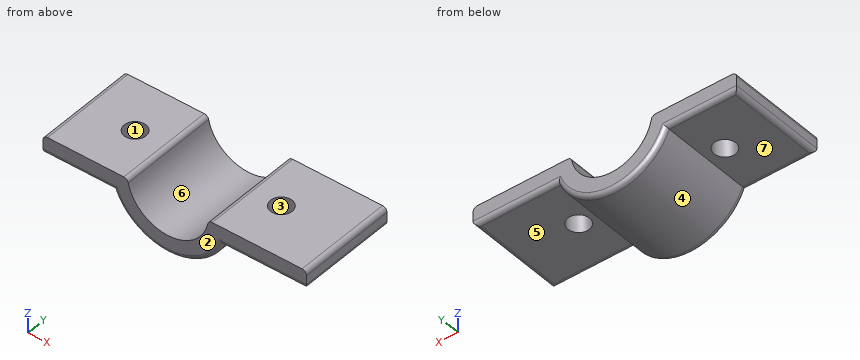
from build123d import *

# Parameters (mm, degrees)
BOSS_EXTRUDE1_DEPTH = 11
SKETCH2_R           = 1.2
CUT_EXTRUDE1_DEPTH  = 2
FILLET1_R           = 0.5


with BuildPart() as part:
    # Sketch1 → Boss-Extrude1 (new body)
    with BuildSketch(Plane(origin=(0, 0, 0), x_dir=(1, 0, 0), z_dir=(0, 1, 0))):
        with BuildLine():
            Line((6, 2.5), (15.35, 2.5))
            Line((15.35, 2.5), (15.35, 0.5))
            Line((15.35, 0.5), (6.480740698, 0.5))
            Line((6.480740698, 0.5), (4.472135955, 0.5))
            ThreePointArc((4.472135955, 0.5), (0, 4.5), (-4.472135955, 0.5))
            Line((-4.472135955, 0.5), (-6.480740698, 0.5))
            Line((-6.480740698, 0.5), (-13.85, 0.5))
            Line((-13.85, 0.5), (-13.85, 2.5))
            Line((-13.85, 2.5), (-6, 2.5))
            ThreePointArc((-6, 2.5), (0, 6.5), (6, 2.5))
        make_face()
    extrude(amount=BOSS_EXTRUDE1_DEPTH)

    # Sketch2 → Cut-Extrude1 (cut)
    with BuildSketch(Plane(origin=(0, 0, -2.5), x_dir=(-1, 0, 0), z_dir=(0, 0, -1))):
        with Locations((-8.1, 5.5)):
            Circle(SKETCH2_R)
        with Locations((8.1, 5.5)):
            Circle(SKETCH2_R)
    extrude(amount=-CUT_EXTRUDE1_DEPTH, mode=Mode.SUBTRACT)

    # Fillet1
    fillet1_edges = [part.edges().sort_by_distance(p)[0] for p in [
        (0, 11, -6.5),
        (-9.925, 0, -2.5),
        (0, 0, -6.5),
        (10.675, 0, -2.5),
        (-9.925, 11, -2.5),
        (15.35, 5.5, -2.5),
        (15.35, 5.5, -0.5),
        (4.472135955, 5.5, -0.5),
        (-4.472135955, 5.5, -0.5),
        (-13.85, 5.5, -0.5),
        (-13.85, 5.5, -2.5),
        (10.675, 11, -2.5),
    ]]
    fillet(fillet1_edges, radius=FILLET1_R)


solid = part.part
Can you work these out from the model? Positions are in its coordinate system, mm. Face numbers are marked on the shaded views. A direction names the side the tool comes from. Round coordinates to 2 decimals unless told otherwise and drop trailing zeros. Order: outer loops, then holes, each group sorted by start corner. A loop starts at its lowest first (then second) coordinate and runs counter-clockwise, first axis right, second up. Notation, with made-up numbers: (12.25, 72.5) - (59.25, 72.5) arc R13 ccw to (59.25, 82.5) - close; hole circle Ø3 at (8, 3.5). An arc over 180 degrees is marked (long way). Answer in a Markdown table with one row per item.
(1) Suppose I cut it at B-B, the plane x = 8.1. Please give me the cut outline in (y, z), plus the area to 3 significant figures.
From the geometry:
| item | result |
|---|---|
| outline | (0, -2) arc R0.5 ccw to (0.5, -2.5) - (4.3, -2.5) - (4.3, -0.5) - (0, -0.5) - close; (6.7, -2.5) - (10.5, -2.5) arc R0.5 ccw to (11, -2) - (11, -0.5) - (6.7, -0.5) - close |
| area | 17.1 mm2 |
(2) For P1, Ø3, axis at x = -8.1, y = 5.5, coming from the +Z side; P2, Ø6, axis at x = -11.5, y = 5, coming from the -Z side; P3, Ø2, axis at y = 8, z = -4, coming from the +X side; P4, Ø2, axis at x = 12.5, z = -5, coming from the -Y side, each with a flat end and sliding along its axis, tell me the tip position at first contact or that it passes through.
From the geometry:
| item | result |
|---|---|
| P1 | stops at z = -0.5 |
| P2 | stops at z = -2.5 |
| P3 | stops at x = 5.77 |
| P4 | passes through |
(3) Please list where these lines run through material, in increasing order: L1, parallel to Y at x = -8.1, z = -1.1; L2, parallel to Z at x = 9.75, y = 3.5; L3, parallel to X at y = 3.75, z = -2.75. Write a range as from..to.
From the geometry:
| item | result |
|---|---|
| L1 | y = 0..4.3, 6.7..11 |
| L2 | z = -2.5..-0.5 |
| L3 | x = -5.89..-3.56, 3.56..5.89 |
(4) Which directions (+Z, -Z, +X, -X, +Y, -Y) give clear straight access to the entire face, cutting with the end or side of a thin tool? Please do the marked faces 5, 6 and 7.
From the geometry:
| item | result |
|---|---|
| face 5 | -Z, +X, +Y, -Y |
| face 6 | +Z, +Y, -Y |
| face 7 | -Z, -X, +Y, -Y |
(5) Suppose I cut it at A-A, the plane y = 5.5. Please give me the cut outline in (x, z), plus the area to 3 significant figures.
From the geometry:
| item | result |
|---|---|
| outline | (-13.85, -2) arc R0.5 ccw to (-13.35, -2.5) - (-9.3, -2.5) - (-9.3, -0.5) - (-13.35, -0.5) arc R0.5 ccw to (-13.85, -1) - close; (-6.9, -2.5) - (-6, -2.5) arc R6.5 ccw to (6, -2.5) - (6.9, -2.5) - (6.9, -0.5) - (4.9, -0.5) arc R0.5 ccw to (4.41, -0.9) arc R4.5 cw to (-4.41, -0.9) arc R0.5 ccw to (-4.9, -0.5) - (-6.9, -0.5) - close; (9.3, -2.5) - (14.85, -2.5) arc R0.5 ccw to (15.35, -2) - (15.35, -1) arc R0.5 ccw to (14.85, -0.5) - (9.3, -0.5) - close |
| area | 55.9 mm2 |
(6) If we mould it in two halves opening along X, with no side actions, what happens to the marked faces 1, 2, 3 and 4? For each: released by +X, released by -X, zero draft, split by the parting line, or undercut.
From the geometry:
| item | result |
|---|---|
| face 1 | undercut |
| face 2 | zero draft |
| face 3 | undercut |
| face 4 | split by the parting line |
(7) Suppose I cut it at C-C, the plane y = 2.75. Please give me the cut outline in (x, z).
From the geometry:
| item | result |
|---|---|
| outline | (-13.85, -2) arc R0.5 ccw to (-13.35, -2.5) - (-6, -2.5) arc R6.5 ccw to (6, -2.5) - (14.85, -2.5) arc R0.5 ccw to (15.35, -2) - (15.35, -1) arc R0.5 ccw to (14.85, -0.5) - (4.9, -0.5) arc R0.5 ccw to (4.41, -0.9) arc R4.5 cw to (-4.41, -0.9) arc R0.5 ccw to (-4.9, -0.5) - (-13.35, -0.5) arc R0.5 ccw to (-13.85, -1) - close |
(8) Suppose I cut it at D-D, the plane x = -9. Please give me the cut outline in (y, z), plus the area to 3 significant figures.
From the geometry:
| item | result |
|---|---|
| outline | (0, -2) arc R0.5 ccw to (0.5, -2.5) - (4.71, -2.5) - (4.71, -0.5) - (0, -0.5) - close; (6.29, -2.5) - (10.5, -2.5) arc R0.5 ccw to (11, -2) - (11, -0.5) - (6.29, -0.5) - close |
| area | 18.7 mm2 |
